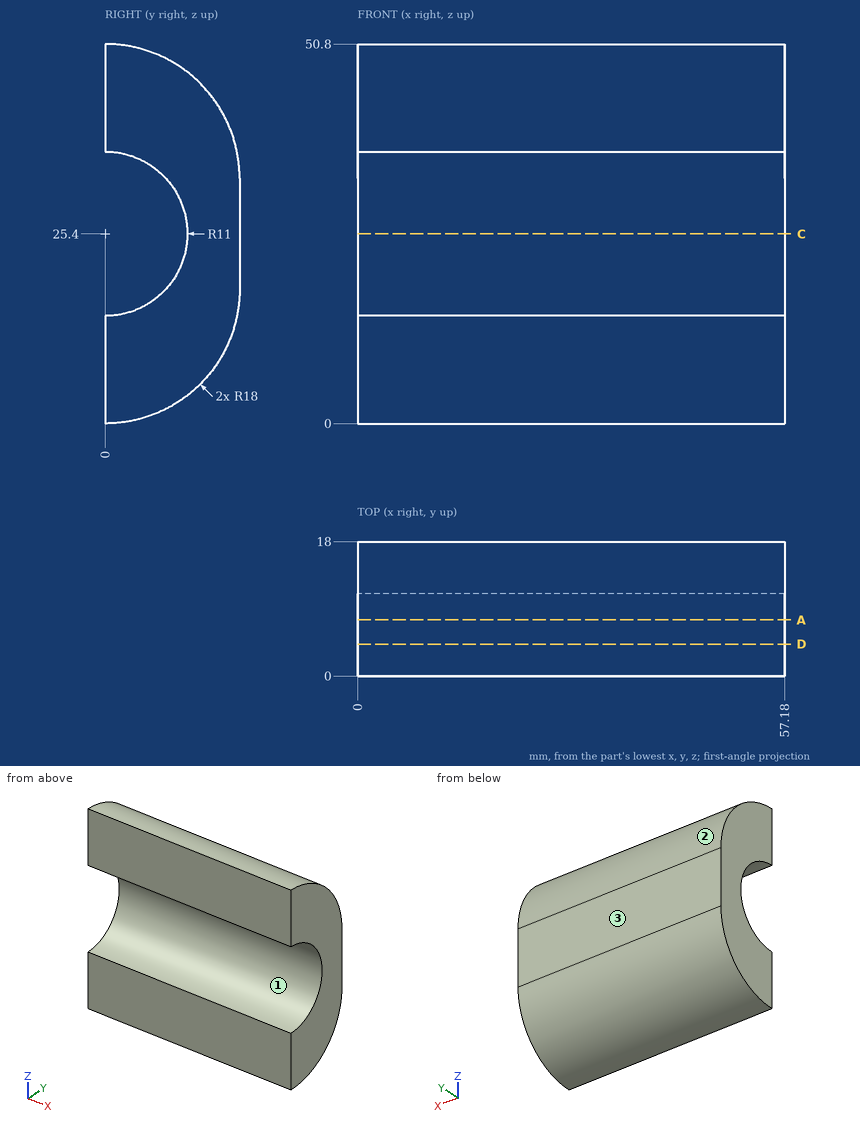
Can you work these out from the drawing? Everything is in mm from the part's minimum corner. Give positions to 0.01 mm unless a question says otherwise; leave off trailing zeros. Loops run counter-clockwise (first coordinate to the right, second up) from the corner with the lowest first, then second, coordinate; pieces in that order, holes last. Notation, with made-up numbers: (-10, 80.5) -> (8, 80.5) arc R30 ccw to (8, 103.5) -> close; hole circle Ø10 at (53.5, -14). An arc over 180 degrees is marked (long way). Put each result on its own line as item: value.
(1) Imagine slicing it at C-C on z = 25.4. Write out the boundary of the cut face in (x, y).
Computed:
outline: (0, 11) -> (57.18, 11) -> (57.18, 18) -> (0, 18) -> close
(2) Imagine slicing it at D-D on y = 4.25. Write out the boundary of the cut face in (x, z).
Computed:
outline: (0, 0.51) -> (57.18, 0.51) -> (57.18, 15.25) -> (0, 15.25) -> close; (0, 35.55) -> (57.18, 35.55) -> (57.18, 50.29) -> (0, 50.29) -> close
(3) Imagine slicing it at A-A on y = 7.5. Write out the boundary of the cut face in (x, z), plus the area to 3 significant figures.
Computed:
outline: (0, 1.64) -> (57.18, 1.64) -> (57.18, 17.35) -> (0, 17.35) -> close; (0, 33.45) -> (57.18, 33.45) -> (57.18, 49.16) -> (0, 49.16) -> close
area: 1,800 mm^2
(4) Thinking about a two-plate mould opening in Z: for the marked faces 1, 2 and 3, which applies, pulls with the +Z half, pulls with the -Z half, needs draft (parallel to the pull), parting line crosses it, or undercut?
Computed:
face 1: undercut
face 2: pulls with the +Z half
face 3: needs draft
(5) I'm going to push flat-ended pins straight in: pin 1 Ø6 at (x, y) = (28, 5.5) entering from +Z; pin 2 Ø5 at (x, y) = (18, 4) entering from +Z; pin 3 Ø10 at (x, y) = (18.5, 13) entering from -Z. Where does each tip first touch, or does it pass through?
Computed:
pin 1: z = 50.63
pin 2: z = 50.74
pin 3: z = 1.88
(6) Please list where these lines run through material, in increasing order: probe 1 along Z at (x, y) = (44.5, 1.5); probe 2 along Z at (x, y) = (24, 5.5); probe 3 along Y at (x, z) = (29.5, 25.5). Write a range as [from, to].
Computed:
probe 1: [0.06, 14.5], [36.3, 50.74]
probe 2: [0.86, 15.87], [34.93, 49.94]
probe 3: [11, 18]
